Verification items for the finished model (mm, model axes). A direction names the side the tool comes from. Give positions to 0.01 mm unless a question says otherwise; leave off trailing zeros. Loops run counter-clockwise (first coordinate to the right, second up) from the corner with the lowest first, then second, coordinate; pieces in that order, holes last. Notation, with made-up numbers: (72.5, -24) -> (111.5, -24) arc R5 cw to (111.5, -20) -> close; hole circle Ø10 at (58, 13.25). An arc over 180 degrees is marked (long way). Answer in a Markdown table with one row per item. Add a question column.
Q1. Release check for a two-part mould opening along X. For faces 1 (the face through (-22.302, 3.451, -12.586)), 2 (the face through (-27, 22, 8)), 3 (the face through (0, 18.2, 2.1)), 4 (the face through (-15, 20, 14)) record: pulls with the +X half, pulls with the -X half, needs draft (parallel to the pull), parting line crosses it, or undercut.
Q2. Material ranges on probe 1 along X at (y, z) = (2.5, -12.5); probe 2 along X at (y, z) = (19.65, 14); probe 3 along Z at (x, y) = (-44.25, 2.25), recorded low to high.
Q3. Section check D-D on y = 19.5. Enter the section's corners in (x, z).
Q4. Set-up check for faces 5 (the face through (-14.449, 3, -12)), 6 (the face through (-28, 20, 20)), 7 (the face through (-34, 3, -20)), 8 (the face through (-35, 7, -13)), 9 (the face through (-27, 18, 10)): record each of +Z, -Z, +X, -X, +Y, -Y from which the full face is reachable in a straight line by a thin tool's end or side.
Q5. Section check A-A on z = 14. Enter the section's corners in (x, y).
Q6. Section check B-B on z = -12.5. Enter the section's corners in (x, y), and give its area (3 significant figures).
Q7. Section check C-C on x = -13.5. Enter the section's corners in (y, z).
Q8. Gauge pin test, flat ends, axial feed: P1, Ø7.5, axis at y = 4, z = -12, coming from the +X side; P2, Ø10, axis at y = 10.5, z = -11.5, coming from the -X side; P3, Ø12, axis at x = -7, y = 5.5, coming from the -Z side; P4, Ø6, axis at x = -23.5, z = 10, coming from the -Y side. Record the tip position at first contact, or that the pin passes through.
Autodesk Inventor part; units mm, degrees
ref_plane "YZ Plane" through (0, 0, 0) normal (1, 0, 0) x (0, 1, 0)
ref_plane "XZ Plane" through (0, 0, 0) normal (0, 1, 0) x (-1, 0, 0)
ref_plane "XY Plane" through (0, 0, 0) normal (0, 0, 1) x (1, 0, 0)
sketch "Эскиз1" plane through (0, 0, 0) normal (0, 1, 0) x (-1, 0, 0)
  circle A0 centre (24.25, -12.5) radius 1.95
  circle A1 centre (44.25, -12.5) radius 1.95
  line L0 (68.5, 0) -> (0, 0)
  line L1 (0, 0) -> (0, -5)
  line L2 (14.449, -5) -> (0, -5)
  line L3 (14.449, -5) -> (14.449, -20)
  line L4 (14.449, -20) -> (54.25, -20)
  line L5 (54.25, -5) -> (54.25, -20)
  line L6 (68.5, -5) -> (54.25, -5)
  line L7 (68.5, 0) -> (68.5, -5)
  point P0 (-5.75, 0)
extrude "Выдавливание1" add sketch "Эскиз1" along normal blind 22
sketch "Эскиз2" plane through (-68.5, 0, 0) normal (0, 0, 1) x (1, 0, 0)
  line L0 (0, 0) -> (0, 22)
  line L1 (0, 22) -> (68.5, 22)
  line L2 (68.5, 0) -> (68.5, 22)
  line L3 (0, 22) -> (68.5, 22)
  line L4 (68.5, 22) -> (68.5, 18)
  line L5 (68.5, 18) -> (0, 18)
  line L6 (0, 18) -> (0, 22)
  dimension "d2" = 4
extrude "Выдавливание2" add sketch "Эскиз2" along normal blind 20
sketch "Эскиз3" plane through (0, 22, 0) normal (0, 1, 0) x (1, 0, 0)
  line L0 (0, 5) -> (-14.449, 5)
  line L1 (-54.25, 20) -> (-14.449, 20)
  line L2 (-14.449, 20) -> (-14.449, 5)
  line L3 (-14.449, 5) -> (-54.25, 5)
  line L4 (-54.25, 5) -> (-54.25, 20)
  point P0 (0, 0)
extrude "Выдавливание3" cut sketch "Эскиз3" against normal blind 15
sketch "Эскиз4" plane through (0, 22, 0) normal (0, 1, 0) x (1, 0, 0)
  line L0 (-68.5, -20) -> (0, -20)
  line L1 (0, -20) -> (-13.5, -20)
  line L2 (-13.5, -20) -> (-13.5, -14)
  line L3 (-13.5, -14) -> (0, -14)
  line L4 (0, -14) -> (0, -20)
  circle A0 centre (-13.5, -14) radius 1.5
  point P0 (0, 0)
  dimension "d7" = 13.5
  dimension "d8" = 6
  dimension "d9" = 3
extrude "Выдавливание4" cut sketch "Эскиз4" against normal blind 15 contours A0 L3 L2 | L2 L3 A0
move faces "Перенос1" translate (14.25, 0, 0) faces at (-68.5, 13.3333, -3.3333)
properties part number "КВ33.044.703 - Стойка оптического датчика оси Y"
Taken from the geometry:
| question | item | result |
|---|---|---|
| 1 | face 1 | undercut |
| 1 | face 2 | needs draft |
| 1 | face 3 | pulls with the +X half |
| 1 | face 4 | undercut |
| 2 | probe 1 | x = -54.25 to -46.2, -42.3 to -26.2, -22.3 to -14.45 |
| 2 | probe 2 | x = -54.25 to -15, -12 to 0 |
| 2 | probe 3 | z = -20 to -14.45, -10.55 to 0 |
| 3 | outline | (-54.25, -5) -> (0, -5) -> (0, 20) -> (-54.25, 20) -> close; hole circle Ø3 at (-13.5, 14) |
| 4 | face 5 | -Z, +X, +Y, -Y |
| 4 | face 6 | +Z, +X, -X, +Y, -Y |
| 4 | face 7 | -Z, +X, -X, +Y, -Y |
| 4 | face 8 | -Z, +X, -X, +Y |
| 4 | face 9 | +Z, +X, -X, -Y |
| 5 | outline | (-54.25, 18) -> (-15, 18) -> (-15, 22) -> (-54.25, 22) -> close; (-12, 18) -> (0, 18) -> (0, 22) -> (-12, 22) -> close |
| 6 | outline | (-54.25, 0) -> (-46.2, 0) -> (-46.2, 7) -> (-54.25, 7) -> close; (-42.3, 0) -> (-26.2, 0) -> (-26.2, 7) -> (-42.3, 7) -> close; (-22.3, 0) -> (-14.45, 0) -> (-14.45, 7) -> (-22.3, 7) -> close |
| 6 | area | 224 mm² |
| 7 | outline | (0, -5) -> (22, -5) -> (22, 12.5) -> (18, 12.5) -> (18, 0) -> (0, 0) -> close; (18, 15.5) -> (22, 15.5) -> (22, 20) -> (18, 20) -> close |
| 8 | P1 | stops at x = -14.45 |
| 8 | P2 | stops at x = -54.25 |
| 8 | P3 | stops at z = -5 |
| 8 | P4 | stops at y = 18 |
